```python
from build123d import *

# Parameters (mm, degrees)
BOSS_EXTRUDE1_DEPTH     = 3
SKETCH3_W               = 42.3
SKETCH3_H               = 30
BOSS_EXTRUDE2_DEPTH     = 3
SKETCH4_R               = 1.1
CUT_EXTRUDE1_DEPTH      = 4
BOSS_EXTRUDE3_DEPTH     = 3
BOSS_EXTRUDE4_START     = -3
SKETCH6_R               = 1.5
BOSS_EXTRUDE4_DEPTH     = 3
MIRROR3_START           = -3
MIRROR3_COPY_1_SKETCH_R = 1.5
MIRROR3_COPY_1_DEPTH    = 3


with BuildPart() as part:
    # Sketch2 → Boss-Extrude1 (new body)
    with BuildSketch(Plane.XY):
        Polygon((-11.75, 3), (11.75, 3), (11.75, 15.6), (21.15, 15.6), (21.15, 0), (-21.15, 0), (-21.15, 15.6), (-11.75, 15.6), align=None)
    extrude(amount=BOSS_EXTRUDE1_DEPTH)

    # Sketch3 → Boss-Extrude2 (add)
    with BuildSketch(Plane.XZ):
        with Locations((0, 15)):
            Rectangle(SKETCH3_W, SKETCH3_H)
    extrude(amount=-BOSS_EXTRUDE2_DEPTH)

    # Sketch4 → Cut-Extrude1 (cut, through all)
    with BuildSketch(Plane.XY.offset(3)):
        with Locations((13.85, 9.55)):
            Circle(SKETCH4_R)
        with Locations((-13.85, 9.55)):
            Circle(SKETCH4_R)
    extrude(amount=-CUT_EXTRUDE1_DEPTH, mode=Mode.SUBTRACT)

    # Sketch5 → Boss-Extrude3 (add)
    with BuildSketch(Plane(origin=(21.15, 0, 0), x_dir=(0, 0, -1), z_dir=(1, 0, 0))):
        Polygon((-3, 15.6), (-13.572655353, 3), (-3, 3), align=None)
    boss_extrude3 = extrude(amount=-BOSS_EXTRUDE3_DEPTH)

    # Mirror1: Boss-Extrude3 across plane
    add(boss_extrude3.mirror(Plane(origin=(0, 0, 0), x_dir=(0, 0, 1), z_dir=(1, 0, 0))))

    # Sketch6 → Boss-Extrude4 (add)
    with BuildSketch(Plane.XZ.offset(BOSS_EXTRUDE4_START)):
        with BuildLine():
            Line((-21.15, 30), (-26.15, 30))
            ThreePointArc((-26.15, 30), (-29.438924173, 27.697070502), (-28.399756634, 23.818844449))
            Line((-28.399756634, 23.818844449), (-21.15, 17.735576331))
            Line((-21.15, 17.735576331), (-21.15, 30))
        make_face()
        with Locations((-26.15, 26.5)):
            Circle(SKETCH6_R, mode=Mode.SUBTRACT)
    boss_extrude4 = extrude(amount=BOSS_EXTRUDE4_DEPTH)

    # Mirror2: Boss-Extrude4 across plane
    add(boss_extrude4.mirror(Plane.XY.offset(15)))

    # Mirror3: Boss-Extrude4 across plane
    add(boss_extrude4.mirror(Plane(origin=(0, 0, 0), x_dir=(0, 0, 1), z_dir=(1, 0, 0))))

    # Mirror3 copy 1 sketch → Mirror3 copy 1 (add)
    with BuildSketch(Plane(origin=(0, 0, 30), x_dir=(-1, 0, 0), z_dir=(0, -1, 0)).offset(MIRROR3_START)):
        with BuildLine():
            Line((-21.15, 30), (-26.15, 30))
            ThreePointArc((-26.15, 30), (-29.438924173, 27.697070502), (-28.399756634, 23.818844449))
            Line((-28.399756634, 23.818844449), (-21.15, 17.735576331))
            Line((-21.15, 17.735576331), (-21.15, 30))
        make_face()
        with Locations((-26.15, 26.5)):
            Circle(MIRROR3_COPY_1_SKETCH_R, mode=Mode.SUBTRACT)
    extrude(amount=MIRROR3_COPY_1_DEPTH)


solid = part.part
```
Model file for the job. Use its own axes, mm. A direction names the side the tool comes from. Coordinates: 2 decimals unless noted, no trailing zeros. Loops run counter-clockwise (first coordinate to the right, second up) from the corner with the lowest first, then second, coordinate; pieces in that order, holes last. Notation, with made-up numbers: (19.5, 17.25) - (44.5, 17.25) arc R24 ccw to (44.5, 43.25) - close; hole circle Ø5 at (29.5, 36). An arc over 180 degrees is marked (long way). Answer as a JSON object with one key per item and string values. Group by question number.
(1) Flat gauge pins, fed straight in: pin 1 (3 mm diameter, centred on y = 6.5, z = 7, fed in from +X); pin 2 (2.5 mm diameter, centred on y = 11, z = 1, fed in from -X); pin 3 (6 mm diameter, centred on x = -23, z = 26, fed in from +Y). Where does each tip first touch, or does it go through?
(2) Cut at A-A (x = -13.85). Give the cut face in (y, z).
(3) Cut at D-D (y = 14.5). Give the cut face in (x, z).
(4) Cut at C-C (y = 9.55). Give the cut face in (x, z).
(5) Cut at B-B (z = 26.5). Give the cut face in (x, y).
(6) Tool access for faces 4 (the face through (-24.8, 1.5, 20.8)), 5 (the face through (-17, 15.6, 1)), 6 (the face through (11.75, 9, 1)): list every direction of +Z, -Z, +X, -X, +Y, -Y with a clear straight run to the whole face (end or side of a thin tool).
(7) Two-plate mould, pull along Y, no slides. Class faces 1 (the face through (-13.99, 10.64, 1.52)), 2 (the face through (-18.15, 7, 6)), 3 (the face through (19.7, 9.4, 8.2)): released by +Y, released by -Y, zero draft, split by the parting line, or undercut.
(8) Probe line 1 along X through (y, z) = (1.5, 3.5); line 2 along Z through (x, y) = (-26.15, 1.9); line 3 along X through (y, z) = (5.5, 2.5). List the from-to ranges inside material, lowest first.
Geometry says:
{
 "1": {"pin 1": "stops at x = 21.15", "pin 2": "stops at x = -21.15", "pin 3": "stops at y = 3"},
 "2": {"outline": "(0, 0) - (8.45, 0) - (8.45, 3) - (3, 3) - (3, 30) - (0, 30) - close; (10.65, 0) - (15.6, 0) - (15.6, 3) - (10.65, 3) - close"},
 "3": {"outline": "(-21.15, 0) - (-11.75, 0) - (-11.75, 3) - (-18.15, 3) - (-18.15, 3.92) - (-21.15, 3.92) - close; (11.75, 0) - (21.15, 0) - (21.15, 3.92) - (18.15, 3.92) - (18.15, 3) - (11.75, 3) - close"},
 "4": {"outline": "(-21.15, 0) - (-14.95, 0) - (-14.95, 3) - (-18.15, 3) - (-18.15, 8.08) - (-21.15, 8.08) - close; (-12.75, 0) - (-11.75, 0) - (-11.75, 3) - (-12.75, 3) - close; (11.75, 0) - (12.75, 0) - (12.75, 3) - (11.75, 3) - close; (14.95, 0) - (21.15, 0) - (21.15, 8.08) - (18.15, 8.08) - (18.15, 3) - (14.95, 3) - close"},
 "5": {"outline": "(-29.65, 0) - (-27.65, 0) - (-27.65, 3) - (-29.65, 3) - close; (-24.65, 0) - (24.65, 0) - (24.65, 3) - (-24.65, 3) - close; (27.65, 0) - (29.65, 0) - (29.65, 3) - (27.65, 3) - close"},
 "6": {"face 4": "-X, +Y, -Y", "face 5": "+Z, -Z, +X, -X, +Y", "face 6": "+Z, -Z, +Y"},
 "7": {"face 1": "undercut", "face 2": "zero draft", "face 3": "released by +Y"},
 "8": {"line 1": "x = -29.65 to -27.65, -24.65 to 24.65, 27.65 to 29.65", "line 2": "z = 0 to 2, 5 to 8.07, 21.93 to 25, 28 to 30", "line 3": "x = -21.15 to -11.75, 11.75 to 21.15"}
}
